```python
from build123d import *

# Parameters (mm, degrees)
F1_DEPTH = 76.2
F2_W     = 27.847374
F2_H     = 51.670779
F3_DEPTH = 50.801
F4_R     = 4.699
F5_DEPTH = 76.2
F6_DEPTH = 19.051


with BuildPart() as f1:
    # F0 (on Right) → F1 (new body)
    with BuildSketch(Plane.YZ):
        Polygon((-19.618108, -25.540555), (-64.068108, -25.540555), (-64.068108, -44.590555), (31.181892, -44.590555), (31.181892, -25.540555), (5.781892, -25.540555), (5.781892, 25.259445), (-19.618108, 25.259445), align=None)
    extrude(amount=F1_DEPTH)

    # F2 (on face) → F3 (cut, through all)
    with BuildSketch(Plane.XZ.offset(19.618108)):
        with Locations((38.1, 25.259445)):
            Rectangle(F2_W, F2_H)
    extrude(amount=-F3_DEPTH, mode=Mode.SUBTRACT)

    # F4 (on face) → F5 (cut)
    with BuildSketch(Plane.XY.offset(-25.540555)):
        with Locations((12.7, -51.368108)):
            Circle(F4_R)
        with Locations((63.5, -51.368108)):
            Circle(F4_R)
        with Locations((10.562182, 18.481892)):
            Circle(F4_R)
        with Locations((61.609245, 18.481892)):
            Circle(F4_R)
    extrude(amount=F5_DEPTH, mode=Mode.SUBTRACT)

    # F4 (on face) → F6 (cut, through all)
    with BuildSketch(Plane.XY.offset(-25.540555)):
        with Locations((12.7, -51.368108)):
            Circle(F4_R)
        with Locations((63.5, -51.368108)):
            Circle(F4_R)
        with Locations((10.562182, 18.481892)):
            Circle(F4_R)
        with Locations((61.609245, 18.481892)):
            Circle(F4_R)
    extrude(amount=-F6_DEPTH, mode=Mode.SUBTRACT)


solid = f1.part
```
The listing builds one solid part. Answer for the finished solid, in the listing's coordinates (mm). A direction names the side the tool comes from. Coordinates: 2 decimals unless noted, no trailing zeros. Loops run counter-clockwise (first coordinate to the right, second up) from the corner with the lowest first, then second, coordinate; pieces in that order, holes last. Notation, with made-up numbers: (26, 32) - (34, 32) arc R13 cw to (34, 47) - close; hole circle Ø6 at (49, 89). An arc over 180 degrees is marked (long way). Write item = value, one per line.
1) Section A-A (z = 9) is taken. Determine the outline of the cut face in (x, y), plus the area to 3 significant figures.
Responses:
outline = (0, -19.62) - (24.18, -19.62) - (24.18, 5.78) - (0, 5.78) - close; (52.02, -19.62) - (76.2, -19.62) - (76.2, 5.78) - (52.02, 5.78) - close
area = 1,230 mm^2
2) Section C-C (y = -3) is taken. Determine the outline of the cut face in (x, z), plus the area to 3 significant figures.
Responses:
outline = (0, -44.59) - (76.2, -44.59) - (76.2, 25.26) - (52.02, 25.26) - (52.02, -0.58) - (24.18, -0.58) - (24.18, 25.26) - (0, 25.26) - close
area = 4,600 mm^2
3) Section B-B (x = 12.7) is taken. Determine the outline of the cut face in (y, z), plus the area to 3 significant figures.
Responses:
outline = (-64.07, -44.59) - (-56.07, -44.59) - (-56.07, -25.54) - (-64.07, -25.54) - close; (-46.67, -44.59) - (14.3, -44.59) - (14.3, -25.54) - (5.78, -25.54) - (5.78, 25.26) - (-19.62, 25.26) - (-19.62, -25.54) - (-46.67, -25.54) - close; (22.67, -44.59) - (31.18, -44.59) - (31.18, -25.54) - (22.67, -25.54) - close
area = 2,770 mm^2
4) Find the intervals of material crossed by line 1 along X through (y, z) = (18.5, -39); line 2 along X through (y, z) = (-16.5, 5); line 3 along Y through (x, z) = (63, -38), in increasing order.
Responses:
line_1 = 0 to 5.86, 15.26 to 56.91, 66.31 to 76.2
line_2 = 0 to 24.18, 52.02 to 76.2
line_3 = -64.07 to -56.04, -46.7 to 13.99, 22.97 to 31.18
5) Section D-D (x = 47.5) is taken. Determine the outline of the cut face in (y, z), plus the area to 3 significant figures.
Responses:
outline = (-64.07, -44.59) - (31.18, -44.59) - (31.18, -25.54) - (5.78, -25.54) - (5.78, -0.58) - (-19.62, -0.58) - (-19.62, -25.54) - (-64.07, -25.54) - close
area = 2,450 mm^2
6) Which of the six approach directions +Z, -Z, +X, -X, +Y, -Y give full straight-line access (tool end or side, diameter ignored) to faces 1 (the face through (24.176, -7, 12)), 2 (the face through (38, 5.782, -6)), 3 (the face through (38, -19.618, -5)), 4 (the face through (38, 31.182, -35))?
Responses:
face_1 = +Z, +Y, -Y
face_2 = +Z, +X, -X, +Y
face_3 = +Z, +X, -X, -Y
face_4 = +Z, -Z, +X, -X, +Y
7) Each of these flat-tipped pins is pushed along its axis until it touches: P1, Ø10, axis at x = 55, z = -12.5, coming from the +Y side; P2, Ø8.5, axis at x = 63.5, y = -51.37, coming from the +Z side; P3, Ø7.5, axis at x = 25.5, y = 20, coming from the +Z side; P4, Ø8, axis at x = 49, z = 8.5, coming from the -Y side. Where does it stop, or does it pass through?
Responses:
P1 = 5.78
P2 = through
P3 = -25.54
P4 = -19.62
